```python
from build123d import *

# Parameters (mm, degrees)
SKETCH1_W                                         = 120
SKETCH1_H                                         = 57.864768683
SKETCH1_R                                         = 2.5
BOSS_EXTRUDE1_DEPTH                               = 7
SKETCH2_W                                         = 54.306051878
SKETCH2_H                                         = 5.719890942
BOSS_EXTRUDE2_DEPTH                               = 87
FILLET1_R                                         = 10
CSK_FOR_0_FLAT_HEAD_MACHINE_SCREW_100_D           = 1.778
CSK_FOR_0_FLAT_HEAD_MACHINE_SCREW_100_CSINK_D     = 3.0226
CSK_FOR_0_FLAT_HEAD_MACHINE_SCREW_100_CSINK_ANGLE = 100


with BuildPart() as part:
    # Sketch1 → Boss-Extrude1 (new body)
    with BuildSketch(Plane.XY):
        with Locations((-0.106761566, 0.160142349)):
            Rectangle(SKETCH1_W, SKETCH1_H)
        with Locations((-44.412811388, 13.398576512)):
            Circle(SKETCH1_R, mode=Mode.SUBTRACT)
        with Locations((43.912956959, 13.468374771)):
            Circle(SKETCH1_R, mode=Mode.SUBTRACT)
    extrude(amount=BOSS_EXTRUDE1_DEPTH)

    # Sketch2 → Boss-Extrude2 (add)
    with BuildSketch(Plane.XY.offset(7)):
        with Locations((-5.436912955, -12.302569894)):
            Rectangle(SKETCH2_W, SKETCH2_H)
    extrude(amount=BOSS_EXTRUDE2_DEPTH)

    # Fillet1
    fillet1_edges = [part.edges().sort_by_distance(p)[0] for p in [
        (-60.106761566, 29.09252669, 3.5),
        (59.893238434, 29.09252669, 3.5),
    ]]
    fillet(fillet1_edges, radius=FILLET1_R)

    # CSK for #0 Flat Head Machine Screw (100)1 (through all)
    with Locations(Plane(origin=(0, -9.442624423, 0), x_dir=(1, 0, 0), z_dir=(0, 1, 0))):
        with Locations((-8.675393381, -34.699580631), (-7.599346026, -45.314885455), (-7.757212548, -55.462997779), (-8.364022161, -66.007770116), (-8.816821696, -79.027415228)):
            CounterSinkHole(CSK_FOR_0_FLAT_HEAD_MACHINE_SCREW_100_D / 2, CSK_FOR_0_FLAT_HEAD_MACHINE_SCREW_100_CSINK_D / 2, counter_sink_angle=CSK_FOR_0_FLAT_HEAD_MACHINE_SCREW_100_CSINK_ANGLE)


solid = part.part
```
Geometry check sheet. Reference: the model listing, model coordinates, mm. A direction names the side the tool comes from. Round coordinates to 2 decimals unless told otherwise and drop trailing zeros. Order: outer loops, then holes, each group sorted by start corner. A loop starts at its lowest first (then second) coordinate and runs counter-clockwise, first axis right, second up. Notation, with made-up numbers: (34.25, 2) -> (57.25, 2) arc R30 ccw to (57.25, 39) -> close; hole circle Ø2 at (-37.5, 43.25). An arc over 180 degrees is marked (long way). Return JSON: item names as keys, results as strings. Group by question number.
Q1. Section check C-C, the plane z = 63. Record the boundary of the cut face in (x, y).
Q2. Tool access check on faces 1 (the flat face through (-32.59, -12, 50)), 2 (the flat face through (59.893, -5, 3)). Record the directions out of +Z, -Z, +X, -X, +Y, -Y that give a thin tool (end or side, any length) a straight path to the whole face; none if there is none.
Q3. Section check A-A, the plane x = 12. Record the boundary of the cut face in (y, z), plus the area to 3 significant figures.
Q4. Release check for a two-part mould opening along Y. For faces 3 (the cylindrical face through (-46.91, 13.51, 3.45)), 4 (the flat face through (21.716, -12, 50)), 5 (the flat face through (-6, -9.443, 50)) record: released by +Y, released by -Y, zero draft, split by the parting line, or undercut.
Q5. Gauge pin test, flat ends, axial feed: pin 1 (4 mm diameter, centred on x = -27, y = 22, fed in from +Z); pin 2 (12 mm diameter, centred on x = -14.5, z = 39, fed in from -Y); pin 3 (2.5 mm diameter, centred on x = -8.82, z = 79.03, fed in from +Y). Record the tip position at first contact, or that the pin passes through.
Q6. Material ranges on probe 1 along Y at (x, z) = (-30.5, 78.5); probe 2 along Z at (x, y) = (19, -24), recorded low to high. Write a range as from..to.
Q7. Section check B-B, the plane y = -5. Record the boundary of the cut face in (x, z).
Numbers:
{
 "1": {"outline": "(-32.59, -15.16) -> (21.72, -15.16) -> (21.72, -9.44) -> (-32.59, -9.44) -> close"},
 "2": {"face 1": "+Z, -X, +Y, -Y", "face 2": "+Z, -Z, +X, +Y, -Y"},
 "3": {"outline": "(-28.77, 0) -> (29.09, 0) -> (29.09, 7) -> (-9.44, 7) -> (-9.44, 94) -> (-15.16, 94) -> (-15.16, 7) -> (-28.77, 7) -> close", "area": "903 mm^2"},
 "4": {"face 3": "undercut", "face 4": "zero draft", "face 5": "released by +Y"},
 "5": {"pin 1": "z = 7", "pin 2": "y = -15.16", "pin 3": "y = -9.66"},
 "6": {"probe 1": "-15.16..-9.44", "probe 2": "0..7"},
 "7": {"outline": "(-60.11, 0) -> (59.89, 0) -> (59.89, 7) -> (-60.11, 7) -> close"}
}
